Autodesk Inventor part; units mm, degrees
ref_plane "YZ Plane" through (0, 0, 0) normal (1, 0, 0) x (0, 1, 0)
ref_plane "XZ Plane" through (0, 0, 0) normal (0, 1, 0) x (-1, 0, 0)
ref_plane "XY Plane" through (0, 0, 0) normal (0, 0, 1) x (1, 0, 0)
sketch "Sketch1" plane through (0, 0, 0) normal (0, 1, 0) x (-1, 0, 0)
  line L0 (8.45, 3.225) -> (-8.45, 3.225)
  line L1 (-8.45, 3.225) -> (-8.45, -3.225)
  line L2 (-8.45, -3.225) -> (8.45, -3.225)
  line L3 (8.45, -3.225) -> (8.45, 3.225)
  point P0 (0, 0)
  dimension "d0" = 16.9
  dimension "d1" = 8.45
  dimension "d2" = 6.45
  dimension "d3" = 3.225
extrude "Extrusion1" add sketch "Sketch1" along normal blind 8.4
sketch "Sketch2" plane through (0, 8.4, 0) normal (0, 1, 0) x (1, 0, 0)
  line L0 (-6.9642, -1.815) -> (7.0758, -1.815)
  line L1 (7.0758, -1.815) -> (7.0758, 2.125)
  line L2 (7.0758, 2.125) -> (-6.9642, 2.125)
  line L3 (-6.9642, 2.125) -> (-6.9642, -1.815)
  line L4 (6.0858, 2.125) -> (-4.7742, 2.125)
  line L5 (-4.7742, 2.125) -> (-4.7742, 2.825)
  line L6 (-4.7742, 2.825) -> (6.0858, 2.825)
  line L7 (6.0858, 2.825) -> (6.0858, 2.125)
  line L8 (-5.1242, -0.825) -> (-3.8742, -0.825)
  line L9 (-3.8742, -0.825) -> (-3.8742, 0.025)
  line L10 (-3.8742, 0.025) -> (5.2858, 0.025)
  line L11 (5.2858, 0.025) -> (5.2858, 1.275)
  line L12 (5.2858, 1.275) -> (-5.1242, 1.275)
  line L13 (-5.1242, 1.275) -> (-5.1242, -0.825)
  line L14 (-8.45, -3.225) -> (8.45, -3.225)
  point P0 (0, 0)
  dimension "d6" = 10.86
  dimension "d7" = 4.5
  dimension "d8" = 1.84
  dimension "d9" = 1.79
  dimension "d10" = 0.8
  dimension "d11" = 10.41
  dimension "d12" = 3.94
  dimension "d13" = 1.55
  dimension "d14" = 1.25
  dimension "d15" = 0.85
  dimension "d16" = 0.85
  dimension "d17" = 1.25
extrude "Extrusion2" cut sketch "Sketch2" against normal blind 4.75
chamfer "Chamfer1" distance 0.2 angle 45 14 edges at (0.0808, 8.4, -1.275) (5.2858, 8.4, -0.65) (0.7058, 8.4, -0.025) (-3.8742, 8.4, 0.4) (-4.4992, 8.4, 0.825) (-5.1242, 8.4, -0.225) (-4.7742, 8.4, -2.475) (-5.8692, 8.4, -2.125) (-6.9642, 8.4, -0.155) (0.0558, 8.4, 1.815) (7.0758, 8.4, -0.155) (6.5808, 8.4, -2.125) (6.0858, 8.4, -2.475) (0.6558, 8.4, -2.825)
sketch "Sketch3" plane through (0, 0, 0) normal (0, -1, 0) x (1, 0, 0)
  line L0 (31.8884, 0.025) -> (-22.6507, 0.025) construction
  line L1 (42.8322, 1.525) -> (-5.5903, 1.525) construction
  circle A0 centre (0, 1.525) radius 0.225
  circle A1 centre (3.81, 1.525) radius 0.225
  circle A2 centre (-3.81, 1.525) radius 0.225
  circle A3 centre (-1.27, 0.025) radius 0.225
  circle A4 centre (-2.54, 0.025) radius 0.225
  circle A5 centre (1.27, 0.025) radius 0.225
  circle A6 centre (2.54, 0.025) radius 0.225
  line L2 (-4.9242, -1.075) -> (5.0858, -1.075)
  line L3 (4.5428, -1.075) -> (-4.5914, -1.075)
  point P0 (0, 0)
  dimension "d23" = 1.27
  dimension "d24" = 1.27
  dimension "d25" = 1.27
  dimension "d26" = 1.27
  dimension "d27" = 1.27
  dimension "d28" = 0
  dimension "d29" = 1.27
  dimension "d30" = 1.5
  dimension "d31" = 0.45
  dimension "d32" = 0.45
  dimension "d33" = 0.45
  dimension "d34" = 0.45
  dimension "d35" = 0.45
  dimension "d36" = 0.45
  dimension "d37" = 0.45
  dimension "d38" = 1.1
extrude "Extrusion3" add sketch "Sketch3" along normal blind 2.85
properties part number "SATA_Conn_TH"
Build history of the part. All positions in model axes, mm. A direction names the side the tool comes from. Give positions to 0.01 mm unless a question says otherwise; leave off trailing zeros. Order: outer loops, then holes, each group sorted by start corner. A loop starts at its lowest first (then second) coordinate and runs counter-clockwise, first axis right, second up. Notation, with made-up numbers: M -9,30.25 L 2,30.25 A21 cw 2,49.25 Z; hole C -39.5,88 d1. An arc over 180 degrees is marked long. Use one line per item in the form item = value.
1) Two-plate mould, pull along Z, no slides. Class faces 3 (the face through (0, 4, -3.225)), 4 (the face through (0.1, 8.4, 2.2)), 5 (the face through (-4.5, 6, 0.825)): released by +Z, released by -Z, zero draft, split by the parting line, or undercut.
Calculated:
face_3 = released by -Z
face_4 = zero draft
face_5 = undercut
2) Saw through at D-D (x = 2.54). Give the cut face in (y, z) (3 decimals).
Calculated:
outline = M -2.85,-0.2 L 0,-0.2 L 0,-3.225 L 8.4,-3.225 L 8.4,-3.025 L 8.2,-2.825 L 3.65,-2.825 L 3.65,-1.275 L 8.2,-1.275 L 8.4,-1.075 L 8.4,-0.225 L 8.2,-0.025 L 3.65,-0.025 L 3.65,1.815 L 8.2,1.815 L 8.4,2.015 L 8.4,3.225 L 0,3.225 L 0,0.25 L -2.85,0.25 Z
3) Tool access for faces 1 (the face through (-5.124, 6, 0)), 2 (the face through (0.2, 8.4, -0.6)): list every direction of +Z, -Z, +X, -X, +Y, -Y with a clear straight run to the whole face (end or side of a thin tool).
Calculated:
face_1 = +Y
face_2 = +Z, -Z, +X, -X, +Y
4) Saw through at B-B (x = -3.25). Give the cut face in (y, z) (3 decimals).
Calculated:
outline = M 0,-3.225 L 8.4,-3.225 L 8.4,-3.025 L 8.2,-2.825 L 3.65,-2.825 L 3.65,-1.275 L 8.2,-1.275 L 8.4,-1.075 L 8.4,-0.225 L 8.2,-0.025 L 3.65,-0.025 L 3.65,1.815 L 8.2,1.815 L 8.4,2.015 L 8.4,3.225 L 0,3.225 Z
5) Drop a flat-ended pin along its axis: pin 1 (3 mm diameter, centred on x = 2, z = 2.5, fed in from -Y). Give the stop position or say it passes through.
Calculated:
pin_1 = 0
6) Saw through at C-C (z = -1.5). Give the cut face in (x, y).
Calculated:
outline = M -8.45,0 L 8.45,0 L 8.45,8.4 L 7.28,8.4 L 7.08,8.2 L 7.08,3.65 L -6.96,3.65 L -6.96,8.2 L -7.16,8.4 L -8.45,8.4 Z
7) Probe probe 1 along X at (y, z) = (3.75, 0.25); probe 2 along Z at (x, y) = (1.25, 4.25) (3 decimals); probe 3 along Z at (x, y) = (5.5, 5.75) (3 decimals). List the from-to ranges inside material, lowest first.
Calculated:
probe_1 = -8.45 to -6.96, -5.12 to -3.87, 7.08 to 8.45
probe_2 = -3.225 to -2.825, -1.275 to -0.025, 1.815 to 3.225
probe_3 = -3.225 to -2.825, 1.815 to 3.225
8) Saw through at A-A (y = 7.25). Give the cut face in (x, z) (3 decimals), plus the area to 3 significant figures.
Calculated:
outline = M -8.45,-3.225 L 8.45,-3.225 L 8.45,3.225 L -8.45,3.225 Z; M -5.124,-1.275 L 5.286,-1.275 L 5.286,-0.025 L -3.874,-0.025 L -3.874,0.825 L -5.124,0.825 Z; hole M -6.964,-2.125 L -4.774,-2.125 L -4.774,-2.825 L 6.086,-2.825 L 6.086,-2.125 L 7.076,-2.125 L 7.076,1.815 L -6.964,1.815 Z
area = 60.2 mm2
